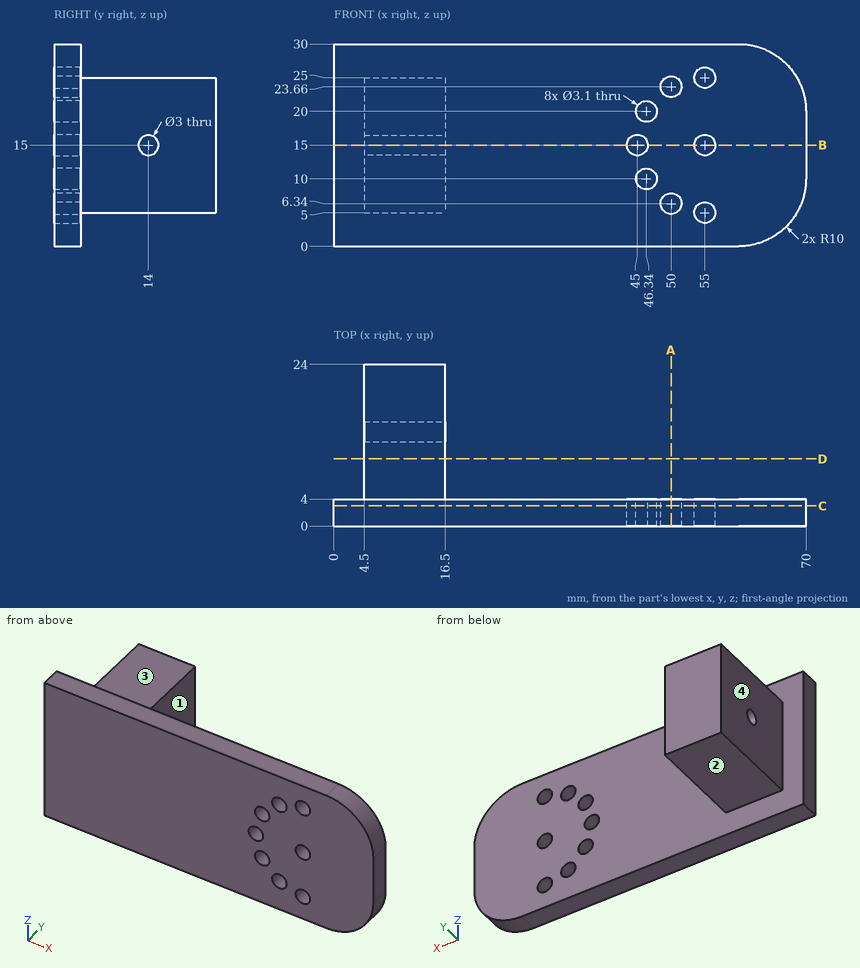
Geometry check sheet. Reference: drawing and pictorial views, mm from the part's lowest x, y, z. A direction names the side the tool comes from. Round coordinates to 2 decimals unless told otherwise and drop trailing zeros. Loops run counter-clockwise (first coordinate to the right, second up) from the corner with the lowest first, then second, coordinate; pieces in that order, holes last. Notation, with made-up numbers: (41.5, 84.25) - (81.5, 84.25) arc R19 cw to (81.5, 111.25) - close; hole circle Ø11 at (50.25, -16). An arc over 180 degrees is marked (long way). Use a Markdown table: item, result.
Q1. Material ranges on line 1 (X direction, y = 3, z = 15); line 2 (X direction, y = 1.85, z = 25); line 3 (X direction, y = 19.75, z = 21), recorded low to high.
Solutions:
| item | result |
|---|---|
| line 1 | x = 0 to 43.45, 46.55 to 53.45, 56.55 to 70 |
| line 2 | x = 0 to 49.22, 50.78 to 53.45, 56.55 to 68.66 |
| line 3 | x = 4.5 to 16.5 |
Q2. Go/stop test with flat-tipped pins: P1, Ø4, axis at x = 55, z = 5, coming from the +Y side; P2, Ø5, axis at y = 2.5, z = 8, coming from the -X side; P3, Ø9.5, axis at x = 9.5, y = 16, coming from the -Z side; P4, Ø2.5, axis at y = 14, z = 15, coming from the -X side. Record where each tip stops, or that it passes through.
Solutions:
| item | result |
|---|---|
| P1 | stops at y = 4 |
| P2 | stops at x = 0 |
| P3 | stops at z = 5 |
| P4 | passes through |
Q3. Access from +Z, -Z, +X, -X, +Y, -Y to the whole of each face (thin tool, end or side, straight path). Record for the marked faces 1, 2, 3 and 4.
Solutions:
| item | result |
|---|---|
| face 1 | +Z, -Z, +X, +Y |
| face 2 | -Z, +X, -X, +Y |
| face 3 | +Z, +X, -X, +Y |
| face 4 | +Z, -Z, -X, +Y |
Q4. Cross-section at A-A on x = 50. Record the cut outline in (y, z).
Solutions:
| item | result |
|---|---|
| outline | (0, 0) - (4, 0) - (4, 4.79) - (0, 4.79) - close; (0, 7.89) - (4, 7.89) - (4, 22.11) - (0, 22.11) - close; (0, 25.21) - (4, 25.21) - (4, 30) - (0, 30) - close |
Q5. Cross-section at D-D on y = 10. Record the cut outline in (x, z), plus the area to 3 significant figures.
Solutions:
| item | result |
|---|---|
| outline | (4.5, 5) - (16.5, 5) - (16.5, 25) - (4.5, 25) - close |
| area | 240 mm2 |
Q6. Cross-section at B-B on z = 15. Record the cut outline in (x, y), plus the area to 3 significant figures.
Solutions:
| item | result |
|---|---|
| outline | (0, 0) - (43.45, 0) - (43.45, 4) - (16.5, 4) - (16.5, 12.5) - (4.5, 12.5) - (4.5, 4) - (0, 4) - close; (4.5, 15.5) - (16.5, 15.5) - (16.5, 24) - (4.5, 24) - close; (46.55, 0) - (53.45, 0) - (53.45, 4) - (46.55, 4) - close; (56.55, 0) - (70, 0) - (70, 4) - (56.55, 4) - close |
| area | 459 mm2 |
Q7. Cross-section at C-C on y = 3. State how many separate pieces and enclosed holes the cut face has, plus the area to 3 significant figures.
Solutions:
| item | result |
|---|---|
| separate pieces | 1 |
| enclosed holes | 8 |
| area | 2,000 mm2 |
